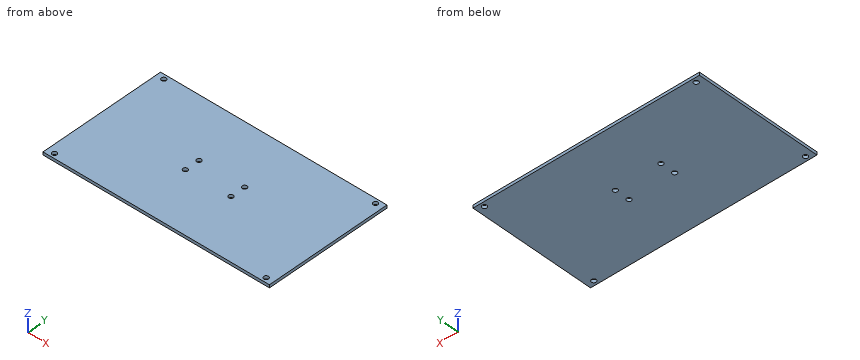
from build123d import *

# Parameters (mm, degrees)
SKETCH_1_W          = 154
SKETCH_1_H          = 86
SKETCH_1_R          = 1.6
EXTRUDE_1_DEPTH     = 2
CUT_EXTRUDE_1_REACH = 183.659
SKETCH_2_R          = 1.6


with BuildPart() as part:
    # 草图1 → 凸台-拉伸1 (new body)
    with BuildSketch(Plane.XY):
        with Locations((-83, 43)):
            Rectangle(SKETCH_1_W, SKETCH_1_H)
        with Locations(Location((-155, 3, 0), (0, 0, 180))):
            Circle(SKETCH_1_R, mode=Mode.SUBTRACT)
        with Locations((-11, 3)):
            Circle(SKETCH_1_R, mode=Mode.SUBTRACT)
        with Locations((-11, 83)):
            Circle(SKETCH_1_R, mode=Mode.SUBTRACT)
        with Locations((-155, 83)):
            Circle(SKETCH_1_R, mode=Mode.SUBTRACT)
    extrude(amount=EXTRUDE_1_DEPTH)

    # 草图2 → 切除-拉伸1 (cut, up to next)
    with BuildSketch(Plane.XY.offset(2), mode=Mode.PRIVATE) as cut_extrude_1_sk1:
        with Locations((-98.5, 48)):
            Circle(SKETCH_2_R)
    cut_extrude_1_tool1 = extrude(cut_extrude_1_sk1.sketch, amount=-CUT_EXTRUDE_1_REACH, mode=Mode.PRIVATE) & part.part
    # 草图2 → 切除-拉伸1 (cut, up to next)
    with BuildSketch(Plane.XY.offset(2), mode=Mode.PRIVATE) as cut_extrude_1_sk2:
        with Locations((-67.5, 48)):
            Circle(SKETCH_2_R)
    cut_extrude_1_tool2 = extrude(cut_extrude_1_sk2.sketch, amount=-CUT_EXTRUDE_1_REACH, mode=Mode.PRIVATE) & part.part
    # 草图2 → 切除-拉伸1 (cut, up to next)
    with BuildSketch(Plane.XY.offset(2), mode=Mode.PRIVATE) as cut_extrude_1_sk3:
        with Locations((-67.5, 38)):
            Circle(SKETCH_2_R)
    cut_extrude_1_tool3 = extrude(cut_extrude_1_sk3.sketch, amount=-CUT_EXTRUDE_1_REACH, mode=Mode.PRIVATE) & part.part
    # 草图2 → 切除-拉伸1 (cut, up to next)
    with BuildSketch(Plane.XY.offset(2), mode=Mode.PRIVATE) as cut_extrude_1_sk4:
        with Locations((-98.5, 38)):
            Circle(SKETCH_2_R)
    cut_extrude_1_tool4 = extrude(cut_extrude_1_sk4.sketch, amount=-CUT_EXTRUDE_1_REACH, mode=Mode.PRIVATE) & part.part
    add(cut_extrude_1_tool1.solids().sort_by_distance((-98.5, 48, 2))[0], mode=Mode.SUBTRACT)
    add(cut_extrude_1_tool2.solids().sort_by_distance((-67.5, 48, 2))[0], mode=Mode.SUBTRACT)
    add(cut_extrude_1_tool3.solids().sort_by_distance((-67.5, 38, 2))[0], mode=Mode.SUBTRACT)
    add(cut_extrude_1_tool4.solids().sort_by_distance((-98.5, 38, 2))[0], mode=Mode.SUBTRACT)


solid = part.part
Geometry: final body of the model. Coordinates: model frame, mm. Coordinates: 2 decimals unless noted, no trailing zeros. Order: outer loops, then holes, each group sorted by start corner. A loop starts at its lowest first (then second) coordinate and runs counter-clockwise, first axis right, second up. Notation, with made-up numbers: M 59,-19 L 111,-19 A13 cw 111,-14 Z; hole C 51.25,-17.75 d2. An arc over 180 degrees is marked long. One line per question, with ' | ' between items. Start each with the question number.
Item 1: Cut plane B-B, the plane y = 48. Return the cut outline in (x, z), then the cut area to 3 significant figures.
Item 2: Cut plane A-A, the plane x = -11. Return the cut outline in (y, z).
Item 3: Ray query, probe 1 along Y at (x, z) = (-98.5, 1.2); probe 2 along Y at (x, z) = (-155, 0.8); probe 3 along X at (y, z) = (47, 0.6). Return the intervals inside material, ascending. Write a range as [from, to].
A:
1) outline: M -160,0 L -100.1,0 L -100.1,2 L -160,2 Z; M -96.9,0 L -69.1,0 L -69.1,2 L -96.9,2 Z; M -65.9,0 L -6,0 L -6,2 L -65.9,2 Z | area: 295 mm2
2) outline: M 0,0 L 1.4,0 L 1.4,2 L 0,2 Z; M 4.6,0 L 81.4,0 L 81.4,2 L 4.6,2 Z; M 84.6,0 L 86,0 L 86,2 L 84.6,2 Z
3) probe 1: y = [0, 36.4], [39.6, 46.4], [49.6, 86] | probe 2: y = [0, 1.4], [4.6, 81.4], [84.6, 86] | probe 3: x = [-160, -99.75], [-97.25, -68.75], [-66.25, -6]
